The listing builds one solid part. Answer for the finished solid, in the listing's coordinates (mm). Face numbers are marked on the shaded views. A direction names the side the tool comes from. Give positions to 0.01 mm unless a question says otherwise; leave off trailing zeros. Loops run counter-clockwise (first coordinate to the right, second up) from the corner with the lowest first, then second, coordinate; pieces in that order, holes last.
Item 1: Section A-A, the plane z = 17.25 is taken. Give the vertices of the cut face in (x, y) (3 decimals).
Item 2: The mould has two halves that part along X. Classify the marked faces 5, 6, 7 and 8: pulls with the +X half, pulls with the -X half, needs draft (parallel to the pull), parting line crosses it, or undercut.
Item 3: Each of these flat-tipped pins is pushed along its axis until it touches: pin 1 Ø6.5 at (x, z) = (40.5, 16) entering from -Y; pin 2 Ø2 at (x, y) = (44.5, 53.5) entering from -Z; pin 3 Ø1.8 at (y, z) = (40, 0) entering from +X. Where does it stop, or does it pass through?
Item 4: Section C-C, the plane y = 50 is taken. Give the vertices of the cut face in (x, z), and give its area (3 significant figures).
Item 5: A tool of negligible diameter and unlimited length cuts with its end or side. For the marked faces 1, 2, 3 and 4, from which of +Z, -Z, +X, -X, +Y, -Y can it reach the whole face along a straight path? Write none if from no direction.
Item 6: Section B-B, the plane x = 39.5 is taken. Give the vertices of the cut face in (y, z).
Item 7: Section D-D, the plane z = 9.75 is taken. Give the vertices of the cut face in (x, y), and give its area (3 significant figures).
Item 8: Consider line 1 along X through (y, z) = (50.5, 15.25); line 2 along Y through (x, z) = (43.75, 14.25); line 3 along Z through (x, y) = (37, 42.5). Determine where each line is inside the solid, lowest interval first.
from build123d import *

# Parameters (mm, degrees)
SKETCH1_W                = 20
SKETCH1_H                = 6
BOSS_EXTRUDE1_DEPTH      = 14
CUT_EXTRUDE1_REACH       = 9.69
SKETCH2_R                = 2.6
SKETCH3_W                = 14
SKETCH3_H                = 20
BOSS_EXTRUDE2_DEPTH      = 3
BOSS_EXTRUDE2_DEPTH_BACK = 3
SKETCH4_R                = 1.025
CUT_EXTRUDE4_DEPTH       = 6
SKETCH5_W                = 5.5
SKETCH5_H                = 8
CUT_EXTRUDE5_DEPTH       = 6
CHAMFER1_SIZE            = 2
CHAMFER2_SIZE            = 2.5
SKETCH6_W                = 5.5
SKETCH6_H                = 0.407228715
CUT_EXTRUDE6_DEPTH       = 2.69
FILLET1_R                = 3


with BuildPart() as part:
    # Sketch1 → Boss-Extrude1 (new body)
    with BuildSketch(Plane(origin=(32.364284334, 0, 0), x_dir=(0, 0, -1), z_dir=(1, 0, 0))):
        with Locations((-7.875866483, 38.765059464)):
            Rectangle(SKETCH1_W, SKETCH1_H)
        with BuildLine():
            Line((-12.22448084, 35.533673821), (-10.765866483, 34.075059464))
            Line((-10.765866483, 34.075059464), (-4.985866483, 34.075059464))
            Line((-4.985866483, 34.075059464), (-3.527252126, 35.533673821))
            ThreePointArc((-3.527252126, 35.533673821), (-3.27095768, 35.704924294), (-2.968637768, 35.765059464))
            Line((-2.968637768, 35.765059464), (-12.783095197, 35.765059464))
            ThreePointArc((-12.783095197, 35.765059464), (-12.480775285, 35.704924294), (-12.22448084, 35.533673821))
        make_face()
    extrude(amount=BOSS_EXTRUDE1_DEPTH)

    # Sketch2 → Cut-Extrude1 (cut, up to next)
    with BuildSketch(Plane.XZ.offset(-34.075059464), mode=Mode.PRIVATE) as cut_extrude1_sk1:
        with Locations((37.864284334, 7.875866483)):
            Circle(SKETCH2_R)
    cut_extrude1_tool1 = extrude(cut_extrude1_sk1.sketch, amount=-CUT_EXTRUDE1_REACH, mode=Mode.PRIVATE) & part.part
    add(cut_extrude1_tool1.solids().sort_by_distance((37.864284, 34.075059, 7.875866))[0], mode=Mode.SUBTRACT)

    # Sketch3 → Boss-Extrude2 (add, two sides)
    with BuildSketch(Plane.XY.offset(17.875866483)) as boss_extrude2_sk:
        with Locations((39.364284334, 45.765059464)):
            Rectangle(SKETCH3_W, SKETCH3_H)
    extrude(amount=BOSS_EXTRUDE2_DEPTH)
    extrude(boss_extrude2_sk.sketch, amount=-BOSS_EXTRUDE2_DEPTH_BACK)

    # Sketch4 → Cut-Extrude4 (cut)
    with BuildSketch(Plane.XY.offset(20.875866483)):
        with Locations((39.364284334, 50.565059464)):
            Circle(SKETCH4_R)
        with Locations((39.364284334, 40.965059464)):
            Circle(SKETCH4_R)
    extrude(amount=-CUT_EXTRUDE4_DEPTH, mode=Mode.SUBTRACT)

    # Sketch5 → Cut-Extrude5 (cut)
    with BuildSketch(Plane(origin=(0, 41.765059464, 0), x_dir=(1, 0, 0), z_dir=(0, 1, 0))):
        with Locations((43.614284334, -1.875866483)):
            Rectangle(SKETCH5_W, SKETCH5_H)
    extrude(amount=-CUT_EXTRUDE5_DEPTH, mode=Mode.SUBTRACT)

    # Chamfer1
    chamfer1_edges = [part.edges().sort_by_distance(p)[0] for p in [
        (40.864284334, 38.765059464, 5.875866483),
    ]]
    chamfer(chamfer1_edges, length=CHAMFER1_SIZE)

    # Chamfer2
    chamfer2_edges = [part.edges().sort_by_distance(p)[0] for p in [
        (44.614284334, 35.765059464, 5.875866483),
    ]]
    chamfer(chamfer2_edges, length=CHAMFER2_SIZE)

    # Sketch6 → Cut-Extrude6 (cut, through all)
    with BuildSketch(Plane(origin=(0, 35.765059464, 0), x_dir=(1, 0, 0), z_dir=(0, 1, 0))):
        with Locations((43.614284334, -3.172252126)):
            Rectangle(SKETCH6_W, SKETCH6_H)
    extrude(amount=-CUT_EXTRUDE6_DEPTH, mode=Mode.SUBTRACT)

    # Fillet1
    fillet1_edges = [part.edges().sort_by_distance(p)[0] for p in [
        (46.364284334, 55.765059464, 17.875866483),
    ]]
    fillet(fillet1_edges, radius=FILLET1_R)


solid = part.part
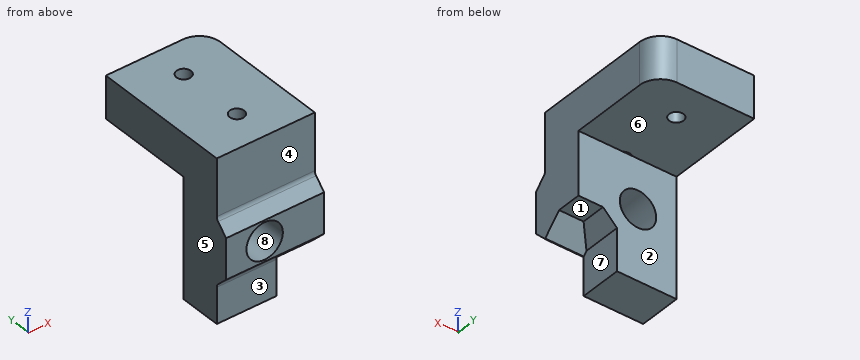
Worked answers:
1. outline: (32.364, 35.765) - (46.364, 35.765) - (46.364, 52.765) arc R3 ccw to (43.364, 55.765) - (32.364, 55.765) - close; hole circle Ø2.05 at (39.364, 40.965); hole circle Ø2.05 at (39.364, 50.565)
2. face 5: pulls with the -X half
2. face 6: needs draft
2. face 7: pulls with the +X half
2. face 8: undercut
3. pin 1: stops at y = 35.76
3. pin 2: stops at z = 14.88
3. pin 3: stops at x = 40.86
4. outline: (32.36, 14.88) - (38.51, 14.88) - (38.51, 20.88) - (32.36, 20.88) - close; (40.22, 14.88) - (46.36, 14.88) - (46.36, 20.88) - (40.22, 20.88) - close
4. area: 73.7 mm2
5. face 1: -Z, +X, +Y
5. face 2: -Z, +X, -X, +Y
5. face 3: -Z, +X, -X, -Y
5. face 4: +Z, +X, -X, -Y
6. outline: (34.08, 4.99) - (35.53, 3.53) arc R0.79 cw to (35.77, 2.97) - (35.77, -2.12) - (41.77, -2.12) - (41.77, 5.85) - (34.08, 5.85) - close; (34.08, 9.9) - (41.77, 9.9) - (41.77, 14.88) - (39.95, 14.88) - (39.95, 20.88) - (35.77, 20.88) - (35.77, 12.78) arc R0.79 cw to (35.53, 12.22) - (34.08, 10.77) - close; (41.98, 14.88) - (49.55, 14.88) - (49.55, 20.88) - (41.98, 20.88) - close; (51.58, 14.88) - (55.77, 14.88) - (55.77, 20.88) - (51.58, 20.88) - close
7. outline: (32.36, 34.08) - (36.06, 34.08) - (36.06, 41.77) - (32.36, 41.77) - close; (39.67, 34.08) - (46.36, 34.08) - (46.36, 41.77) - (39.67, 41.77) - close
7. area: 79.9 mm2
8. line 1: x = 32.36 to 38.34, 40.39 to 46.36
8. line 2: y = 35.77 to 41.77
8. line 3: z = 14.88 to 20.88
